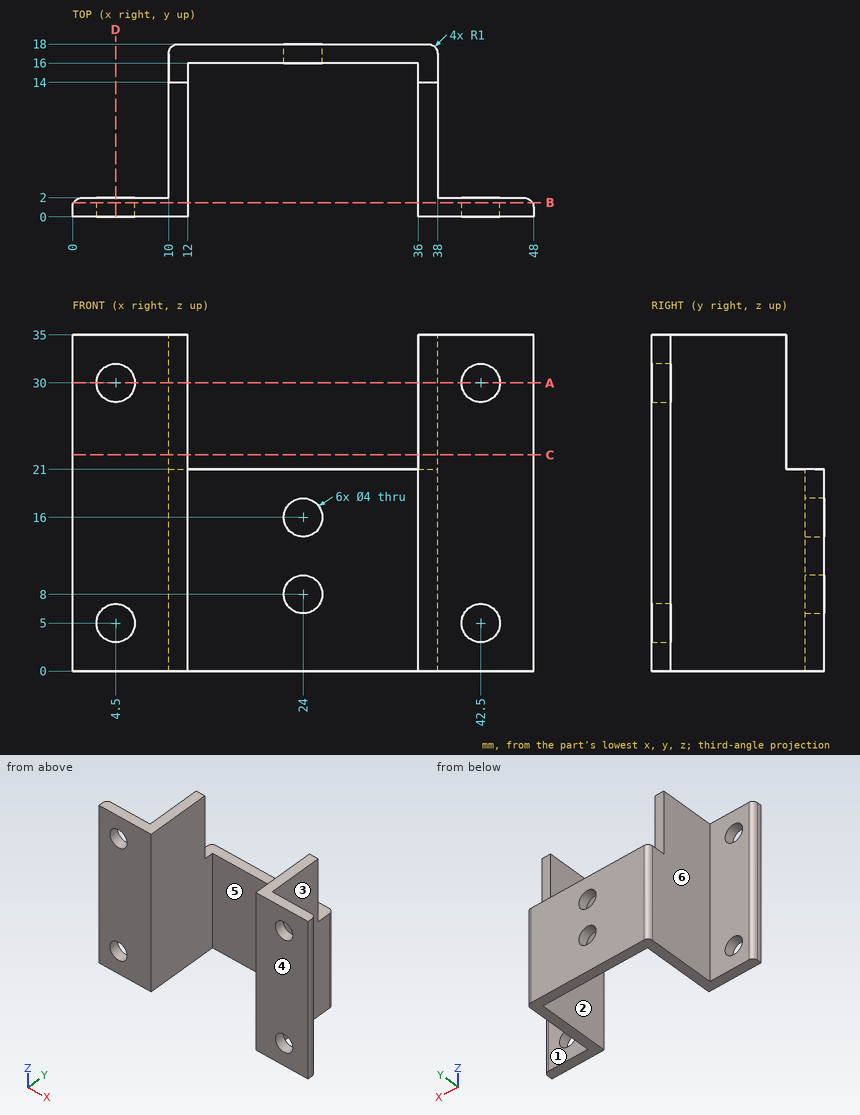
Input: dimensioned drawing with shaded views. Units: mm. Origin: part minimum x, y, z. A direction names the side the tool comes from. Coordinates: 2 decimals unless noted, no trailing zeros. Loops run counter-clockwise (first coordinate to the right, second up) from the corner with the lowest first, then second, coordinate; pieces in that order, holes last. Notation, with made-up numbers: M 26.25,50 L 71.25,50 A29 cw 71.25,89 Z; hole C -3.75,49 d5. An arc over 180 degrees is marked long. Use a Markdown table: item, result. Add a question column.
1) Set-up query: the marked faces 4, 5 and 6. Return all of +Z, -Z, +X, -X, +Y, -Y with unobstructed straight access to the full face (end or side cutting, diameter ignored); none if empty.
2) Line query: L1, parallel to X at y = 1.05, z = 5; L2, parallel to X at y = 5.75, z = 32.5; L3, parallel to Y at x = 27.5, z = 17. Output: solid intervals per line, ascending. Write a range as from..to.
3) Section A-A, the plane z = 30. Return the cut outline in (x, y), plus the area to 3 significant figures.
4) Draft query along X for the marked faces 1, 2 and 3. Return one class per face: +X half, -X half, draft (parallel to the pull), parting line (faces both ways), or undercut.
5) Section B-B, the plane y = 1.5. Return the cut outline in (x, z).
6) Pin query (flat end, axial travel): P1, Ø12, axis at x = 15, z = 26.5, coming from the +Y side; P2, Ø1, axis at x = 11, z = 29, coming from the +Y side; P3, Ø4.5, axis at y = 13, z = 17.5, coming from the -X side; P4, Ø2, axis at x = 23.5, y = 16, coming from the +Z side. Return the tip coordinate at first contact, or that it passes through.
7) Section C-C, the plane z = 22.5. Return the cut outline in (x, y), plus the area to 3 significant figures.
8) Section D-D, the plane x = 4.5. Return the cut outline in (y, z).
Answer below:
| question | item | result |
|---|---|---|
| 1 | face 4 | +Z, -Z, +X, -X, -Y |
| 1 | face 5 | +Z, -Z, -Y |
| 1 | face 6 | +Z, -Z, -X, +Y |
| 2 | L1 | 0..2.5, 6.5..12, 36..40.5, 44.5..48 |
| 2 | L2 | 10..12, 36..38 |
| 2 | L3 | 16..18 |
| 3 | outline | M 0,0 L 2.5,0 L 2.5,2 L 1,2 A1 ccw 0,1 Z; M 6.5,0 L 12,0 L 12,14 L 10,14 L 10,2 L 6.5,2 Z; M 36,0 L 40.5,0 L 40.5,2 L 38,2 L 38,14 L 36,14 Z; M 44.5,0 L 48,0 L 48,1 A1 ccw 47,2 L 44.5,2 Z |
| 3 | area | 79.6 mm2 |
| 4 | face 1 | draft |
| 4 | face 2 | undercut |
| 4 | face 3 | +X half |
| 5 | outline | M 0.13,0 L 12,0 L 12,35 L 0.13,35 Z; M 36,0 L 47.87,0 L 47.87,35 L 36,35 Z; hole C 4.5,5 d4; hole C 4.5,30 d4; hole C 42.5,5 d4; hole C 42.5,30 d4 |
| 6 | P1 | y = 18 |
| 6 | P2 | y = 14 |
| 6 | P3 | x = 10 |
| 6 | P4 | z = 21 |
| 7 | outline | M 0,0 L 12,0 L 12,14 L 10,14 L 10,2 L 1,2 A1 ccw 0,1 Z; M 36,0 L 48,0 L 48,1 A1 ccw 47,2 L 38,2 L 38,14 L 36,14 Z |
| 7 | area | 95.6 mm2 |
| 8 | outline | M 0,0 L 2,0 L 2,3 L 0,3 Z; M 0,7 L 2,7 L 2,28 L 0,28 Z; M 0,32 L 2,32 L 2,35 L 0,35 Z |
